Can you work these out from the model? Positions are in its coordinate system, mm. A direction names the side the tool comes from. Coordinates: 2 decimals unless noted, no trailing zeros. Order: outer loops, then holes, each group sorted by start corner. A loop starts at its lowest first (then second) coordinate and runs counter-clockwise, first axis right, second up. Notation, with made-up numbers: (61, 13.25) -> (116, 13.25) arc R5 ccw to (116, 20.25) -> close; hole circle Ø10 at (28, 20.5). An arc over 180 degrees is marked (long way). Answer in a Markdown table with one row per item. Add a question column.
1. Imagine slicing it at A-A on x = 8.5. Write out the boundary of the cut face in (y, z) (3 decimals).
2. Imagine slicing it at B-B on z = 2.3. State how many separate pieces and enclosed holes the cut face has, plus the area to 3 significant figures.
3. If I drill on line 1 along Y through (x, z) = (3.5, 1.4); line 2 along Y through (x, z) = (22.5, 0.5); line 3 along X through (y, z) = (-31, 2.6), over which ranges is the centre line in solid material (lowest first)? Write a range as [from, to].
4. Will these pins go through, and if not, where does the flat tip stop? pin 1 (1.3 mm diameter, centred on x = -1.21, y = -5.2, fed in from +Z); pin 2 (2 mm diameter, centred on x = 12.5, y = 2, fed in from -Z); pin 3 (1 mm diameter, centred on x = -2, z = 1.5, fed in from +Y); pin 4 (1.6 mm diameter, centred on y = 5, z = 2, fed in from +X).
5. We'd pull the mould along Y, two halves only. Please class faces 3 (the face through (12, -38.1, 2)), 4 (the face through (31.406, -0.301, 1.61)), 5 (the face through (20, 5, 2)), 6 (the face through (12, -5.2, 2)): pulls with the +Y half, pulls with the -Y half, needs draft (parallel to the pull), parting line crosses it, or undercut.
6. On a 3-axis mill with a long thin cutter (end or side, diameter ignored), from which of +Z, -Z, +X, -X, +Y, -Y can I reach the whole of each face in a straight line? I mean faces 1 (the face through (-0.301, 0.285, 1.61)), 2 (the face through (0.05, -6.487, 1.565)). Say none if no direction works.
7. Imagine slicing it at C-C on x = 16.5. Write out the boundary of the cut face in (y, z) (3 decimals), plus the area to 3 significant figures.
from build123d import *

# Parameters (mm, degrees)
SKETCH1_R           = 0.8
SKETCH1_R_2         = 1.25
BOSS_EXTRUDE1_DEPTH = 3.175
FILLET1_R           = 1


with BuildPart() as part:
    # Sketch1 → Boss-Extrude1 (new body)
    with BuildSketch(Plane.XY):
        Polygon((31.690894529, -38.1), (31.690894529, 0), (20, 0), (20, 10.87553853), (0, 10.87553853), (0, 0), (-6.409105471, 0), (-6.409105471, -38.1), align=None)
        with Locations((26.490894529, -32.9)):
            Circle(SKETCH1_R, mode=Mode.SUBTRACT)
        with Locations((-1.209105471, -32.9)):
            Circle(SKETCH1_R, mode=Mode.SUBTRACT)
        with Locations((-1.209105471, -5.2)):
            Circle(SKETCH1_R, mode=Mode.SUBTRACT)
        with Locations((26.490894529, -5.2)):
            Circle(SKETCH1_R, mode=Mode.SUBTRACT)
        with Locations((16.335044769, 3.811593223)):
            Circle(SKETCH1_R_2, mode=Mode.SUBTRACT)
        with Locations((3.664955231, 3.811593223)):
            Circle(SKETCH1_R_2, mode=Mode.SUBTRACT)
        with BuildLine():
            Line((26.490894529, -7), (26.490894529, -31.1))
            ThreePointArc((26.490894529, -31.1), (25.218102323, -31.627207794), (24.690894529, -32.9))
            Line((24.690894529, -32.9), (0.590894529, -32.9))
            ThreePointArc((0.590894529, -32.9), (0.063686735, -31.627207794), (-1.209105471, -31.1))
            Line((-1.209105471, -31.1), (-1.209105471, -7))
            ThreePointArc((-1.209105471, -7), (0.063686735, -6.472792206), (0.590894529, -5.2))
            Line((0.590894529, -5.2), (24.690894529, -5.2))
            ThreePointArc((24.690894529, -5.2), (25.218102323, -6.472792206), (26.490894529, -7))
        make_face(mode=Mode.SUBTRACT)
    extrude(amount=BOSS_EXTRUDE1_DEPTH)

    # Fillet1
    fillet1_edges = [part.edges().sort_by_distance(p)[0] for p in [
        (20, 10.87553853, 1.5875),
        (20, 0, 1.5875),
        (31.690894529, 0, 1.5875),
        (31.690894529, -38.1, 1.5875),
        (-6.409105471, -38.1, 1.5875),
        (-6.409105471, 0, 1.5875),
        (0, 0, 1.5875),
        (0, 10.87553853, 1.5875),
    ]]
    fillet(fillet1_edges, radius=FILLET1_R)


solid = part.part
Answers follow:
| question | item | result |
|---|---|---|
| 1 | outline | (-38.1, 0) -> (-32.9, 0) -> (-32.9, 3.175) -> (-38.1, 3.175) -> close; (-5.2, 0) -> (10.876, 0) -> (10.876, 3.175) -> (-5.2, 3.175) -> close |
| 2 | separate pieces | 1 |
| 2 | enclosed holes | 7 |
| 2 | area | 893 mm² |
| 3 | line 1 | y = [-38.1, -32.9], [-5.2, 2.57], [5.05, 10.88] |
| 3 | line 2 | y = [-38.1, -32.9], [-5.2, 0] |
| 3 | line 3 | x = [-6.41, -1.21], [26.49, 31.69] |
| 4 | pin 1 | passes through |
| 4 | pin 2 | stops at z = 0 |
| 4 | pin 3 | stops at y = 0 |
| 4 | pin 4 | stops at x = 20 |
| 5 | face 3 | pulls with the -Y half |
| 5 | face 4 | pulls with the +Y half |
| 5 | face 5 | needs draft |
| 5 | face 6 | undercut |
| 6 | face 1 | +Z, -Z, -X, +Y |
| 6 | face 2 | +Z, -Z |
| 7 | outline | (-38.1, 0) -> (-32.9, 0) -> (-32.9, 3.175) -> (-38.1, 3.175) -> close; (-5.2, 0) -> (2.573, 0) -> (2.573, 3.175) -> (-5.2, 3.175) -> close; (5.051, 0) -> (10.876, 0) -> (10.876, 3.175) -> (5.051, 3.175) -> close |
| 7 | area | 59.7 mm² |
